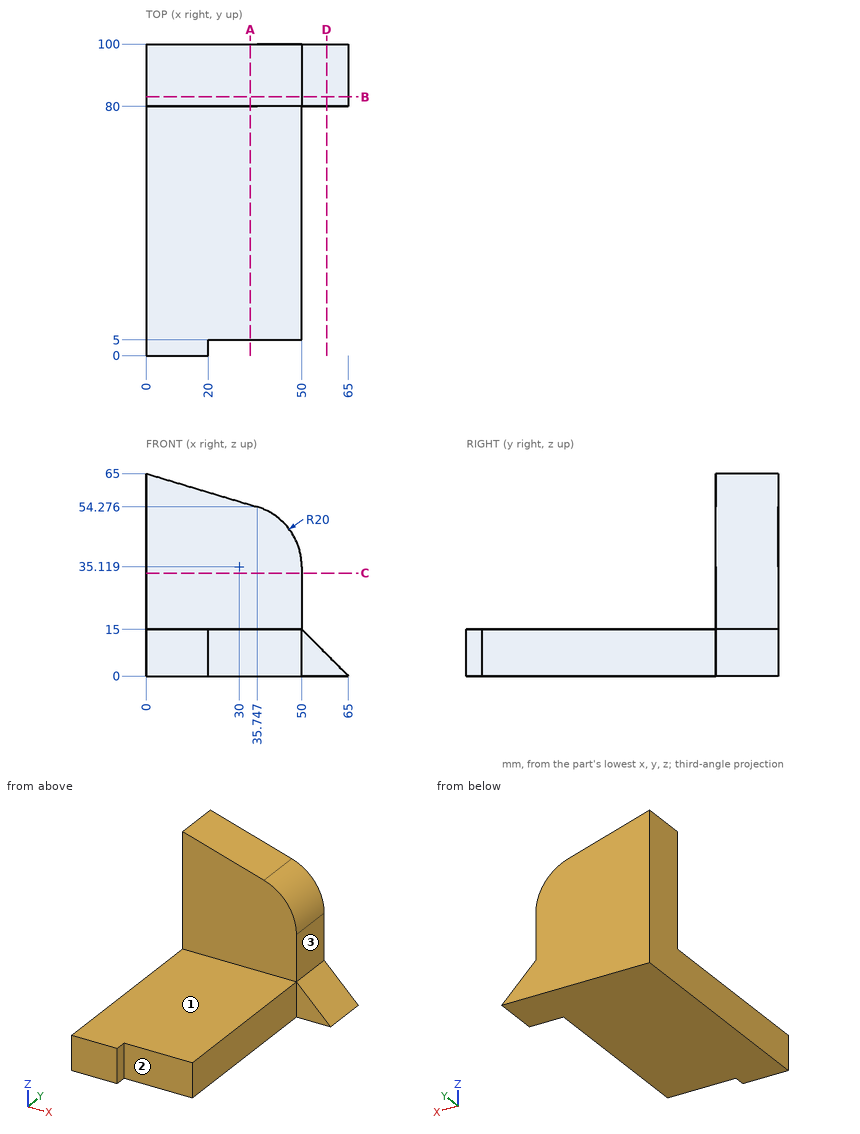
Print and shaded views of the part. All mm, measured from the part's lowest x, y and z. A direction names the side the tool comes from. Coordinates: 2 decimals unless noted, no trailing zeros. Order: outer loops, then holes, each group sorted by start corner. A loop starts at its lowest first (then second) coordinate and runs counter-clockwise, first axis right, second up. Notation, with made-up numbers: M 10,-3.5 L 31,-3.5 A33 cw 31,29.5 Z; hole C -24,77 d6. An arc over 180 degrees is marked long. Write each question's results on one line, items separated by ' | '. Start each with the question number.
Q1. Cut at C-C (z = 33). List the corners of the cut face in (x, y), then the cut area to 3 significant figures.
Q2. Cut at B-B (y = 83). List the corners of the cut face in (x, z).
Q3. Flat gauge pins, fed straight in: P1, Ø2, axis at x = 25.5, z = 51, coming from the -Y side; P2, Ø2.5, axis at y = 3, z = 10, coming from the +X side; P3, Ø16.5, axis at y = 44.5, z = 4, coming from the +X side. Where does each tip first touch, or does it go through?
Q4. Cut at A-A (x = 33.5). List the corners of the cut face in (y, z).
Q5. Which spindle directions (+Z, -Z, +X, -X, +Y, -Y) get a long thin tool onto all of the face, cutting with end or side? Do the marked faces 1, 2 and 3. Say none if no direction does.
Q6. Cut at D-D (x = 58). List the corners of the cut face in (y, z).
Q7. Drill centre lines: probe 1 along Z at (x, y) = (27, 17); probe 2 along Y at (x, z) = (34.5, 37); probe 3 along Y at (x, z) = (36, 8.5). Where is each one in solid material? Low to high. Write a range as from..to.
Found:
1) outline: M 0,80 L 50,80 L 50,100 L 0,100 Z | area: 1,000 mm²
2) outline: M 0,0 L 65,0 L 50,15 L 50,35.12 A20 ccw 35.75,54.28 L 0,65 Z
3) P1: y = 80 | P2: x = 20 | P3: x = 50
4) outline: M 5,0 L 100,0 L 100,54.95 L 80,54.95 L 80,15 L 5,15 Z
5) face 1: +Z, +X, -X, -Y | face 2: +Z, -Z, +X, -Y | face 3: +Z, +X, +Y, -Y
6) outline: M 80,0 L 100,0 L 100,7 L 80,7 Z
7) probe 1: 0..15 | probe 2: 80..100 | probe 3: 5..100
